Work out the finished part from the listing and answer in its coordinate system (mm). Face numbers are marked on the shaded views. A direction names the side the tool comes from. Round coordinates to 2 decimals unless told otherwise and drop trailing zeros. Write each loop counter-clockwise with the first axis right and the second up, starting at its lowest first coordinate (ties: lowest second). Pieces come first, ordered by that corner, then holes. Notation, with made-up numbers: (37, -14.5) -> (83, -14.5) arc R13 cw to (83, 5.5) -> close; hole circle Ø3 at (70.5, -18). An arc over 180 degrees is marked (long way). One line per question, with ' | ' between items. Start each with the question number.
```python
from build123d import *

# Parameters (mm, degrees)
SKETCH_1_W             = 51
SKETCH_1_H             = 25
SKETCH_1_W_2           = 9
SKETCH_1_H_2           = 6.5
EXTRUDE_1_DEPTH        = 9
SKETCH_2_W             = 51
SKETCH_2_H             = 20
CUT_EXTRUDE_1_DEPTH    = 0.5
SKETCH_3_R             = 0.75
CUT_EXTRUDE_2_DEPTH    = 31.336652749
PATTERN_LINEAR_1_COUNT = 4
PATTERN_LINEAR_1_PITCH = 12
SKETCH_4_W             = 45
SKETCH_4_H             = 6.5
CUT_EXTRUDE_3_DEPTH    = 30.643717716


with BuildPart() as part:
    # 草图1 → 凸台-拉伸1 (new body)
    with BuildSketch(Plane(origin=(0, 0, 0), x_dir=(1, 0, 0), z_dir=(0, 1, 0))):
        Rectangle(SKETCH_1_W, SKETCH_1_H)
        with Locations((-18, 4.5)):
            Rectangle(SKETCH_1_W_2, SKETCH_1_H_2, mode=Mode.SUBTRACT)
        with Locations((-18, -4.5)):
            Rectangle(SKETCH_1_W_2, SKETCH_1_H_2, mode=Mode.SUBTRACT)
        with Locations((-6, 4.5)):
            Rectangle(SKETCH_1_W_2, SKETCH_1_H_2, mode=Mode.SUBTRACT)
        with Locations((-6, -4.5)):
            Rectangle(SKETCH_1_W_2, SKETCH_1_H_2, mode=Mode.SUBTRACT)
        with Locations((6, 4.5)):
            Rectangle(SKETCH_1_W_2, SKETCH_1_H_2, mode=Mode.SUBTRACT)
        with Locations((6, -4.5)):
            Rectangle(SKETCH_1_W_2, SKETCH_1_H_2, mode=Mode.SUBTRACT)
        with Locations((18, 4.5)):
            Rectangle(SKETCH_1_W_2, SKETCH_1_H_2, mode=Mode.SUBTRACT)
        with Locations((18, -4.5)):
            Rectangle(SKETCH_1_W_2, SKETCH_1_H_2, mode=Mode.SUBTRACT)
    extrude(amount=EXTRUDE_1_DEPTH)

    # 草图2 → 切除-拉伸1 (cut)
    with BuildSketch(Plane(origin=(0, 9, 0), x_dir=(1, 0, 0), z_dir=(0, 1, 0))):
        Rectangle(SKETCH_2_W, SKETCH_2_H)
    extrude(amount=-CUT_EXTRUDE_1_DEPTH, mode=Mode.SUBTRACT)

    # 草图3 → 切除-拉伸2 (cut, symmetric)
    with BuildSketch(Plane.XY.offset(1.25)):
        with Locations((-18, 4.9)):
            Circle(SKETCH_3_R)
    cut_extrude_2 = extrude(amount=CUT_EXTRUDE_2_DEPTH, both=True, mode=Mode.SUBTRACT)

    # 阵列(线性)1: 切除-拉伸2 ×4
    with Locations(*[(i * PATTERN_LINEAR_1_PITCH, 0, 0) for i in range(1, PATTERN_LINEAR_1_COUNT)]):
        add(cut_extrude_2, mode=Mode.SUBTRACT)

    # 草图4 → 切除-拉伸3 (cut, through all)
    with BuildSketch(Plane(origin=(0, 8.5, 0), x_dir=(1, 0, 0), z_dir=(0, 1, 0))):
        with Locations((0, 4.5)):
            Rectangle(SKETCH_4_W, SKETCH_4_H)
        with Locations((0, -4.5)):
            Rectangle(SKETCH_4_W, SKETCH_4_H)
    extrude(amount=-CUT_EXTRUDE_3_DEPTH, mode=Mode.SUBTRACT)


solid = part.part
```
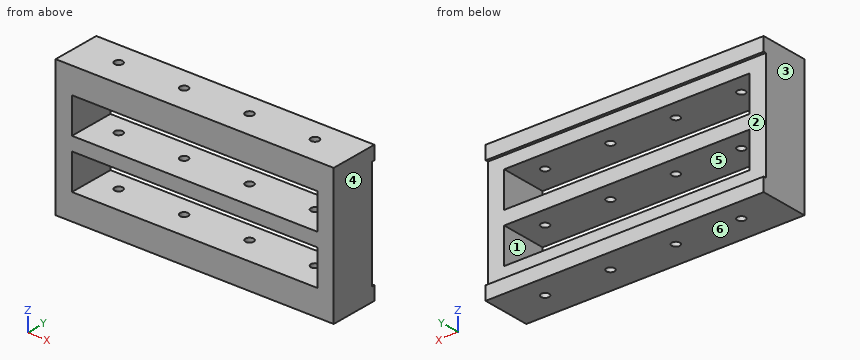
(1) For the marked faces 1, 2 and 3, determine the directions among +Z, -Z, +X, -X, +Y, -Y from which every point of the face is accessible in a straight line to the end or side of a thin tool.
(2) Consider L1, parallel to Z at x = 20.5, y = 4.25; L2, parallel to X at y = 3.25, z = 6; L3, parallel to X at y = 4.75, z = -9.25. Determine where each line is inside the solid, lowest interval first.
(3) Given pin 1 Ø10 at (x, z) = (-10, -0.5) entering from +Y; pin 2 Ø0.9 at (x, y) = (18, 4.9) entering from -Z, each flat-ended and moving along its own axis, determine where each tip first touches the part or whether it passes through.
(4) A cutting plane is placed at D-D, the plane x = 6. Determine the outline of the cut face in (y, z), then the cut area to 3 significant figures.
(5) A cutting plane is placed at C-C, the plane z = 2. Determine the outline of the cut face in (x, y), then the cut area to 3 significant figures.
(6) A cutting plane is placed at B-B, the plane x = -14. Determine the outline of the cut face in (y, z), then the cut area to 4 significant figures.
(7) The mould has two halves that part along X. Classify the marked faces 4, 5 and 6: +X half, -X half, draft (parallel to the pull), parting line (faces both ways), or undercut.
(8) A cutting plane is placed at A-A, the plane y = 2.75. Determine the outline of the cut face in (x, z), then the cut area to 3 significant figures.
Returned:
1) face 1: +Y, -Y | face 2: +X, -X, +Y | face 3: +Z, -Z, -X, +Y, -Y
2) L1: -12.5 to -7.75, -1.25 to 1.25, 7.75 to 12.5 | L2: -25.5 to -22.5, 22.5 to 25.5 | L3: -25.5 to -18.73, -17.27 to -6.73, -5.27 to 5.27, 6.73 to 17.27, 18.73 to 25.5
3) pin 1: y = 8.5 | pin 2: through
4) outline: (0, -12.5) -> (4.15, -12.5) -> (4.15, -7.75) -> (0, -7.75) -> close; (0, -1.25) -> (4.15, -1.25) -> (4.15, 1.25) -> (0, 1.25) -> close; (0, 7.75) -> (4.15, 7.75) -> (4.15, 12.5) -> (0, 12.5) -> close; (5.65, -12.5) -> (9, -12.5) -> (9, -10) -> (8.5, -10) -> (8.5, -7.75) -> (5.65, -7.75) -> close; (5.65, -1.25) -> (8.5, -1.25) -> (8.5, 1.25) -> (5.65, 1.25) -> close; (5.65, 7.75) -> (8.5, 7.75) -> (8.5, 10) -> (9, 10) -> (9, 12.5) -> (5.65, 12.5) -> close | area: 86.5 mm2
5) outline: (-25.5, 0) -> (-22.5, 0) -> (-22.5, 8.5) -> (-25.5, 8.5) -> close; (22.5, 0) -> (25.5, 0) -> (25.5, 8.5) -> (22.5, 8.5) -> close | area: 51.0 mm2
6) outline: (0, -12.5) -> (9, -12.5) -> (9, -10) -> (8.5, -10) -> (8.5, -7.75) -> (0, -7.75) -> close; (0, -1.25) -> (8.5, -1.25) -> (8.5, 1.25) -> (0, 1.25) -> close; (0, 7.75) -> (8.5, 7.75) -> (8.5, 10) -> (9, 10) -> (9, 12.5) -> (0, 12.5) -> close | area: 104.5 mm2
7) face 4: +X half | face 5: undercut | face 6: draft
8) outline: (-25.5, -12.5) -> (25.5, -12.5) -> (25.5, 12.5) -> (-25.5, 12.5) -> close; hole (-22.5, -7.75) -> (22.5, -7.75) -> (22.5, -1.25) -> (-22.5, -1.25) -> close; hole (-22.5, 1.25) -> (22.5, 1.25) -> (22.5, 7.75) -> (-22.5, 7.75) -> close | area: 690 mm2
